For this review, take the finished solid that the model builds, in its own axes (mm). A direction names the side the tool comes from. Round coordinates to 2 decimals unless told otherwise and drop trailing zeros. Order: outer loops, then holes, each group sorted by start corner. A loop starts at its lowest first (then second) coordinate and runs counter-clockwise, first axis right, second up. Notation, with made-up numbers: (-17.75, 1.5) - (40.25, 1.5) arc R27 cw to (40.25, 40.5) - close; hole circle Ø4 at (68, 16.25). An arc over 180 degrees is marked (long way). Write each question's results on one line, items separated by ' | '. Start each with the question number.
(1) Take a section at A-A, the plane y = 9.5. Give the boundary of the cut face in (x, z), plus the area to 3 significant figures.
(2) Insertion check: pin 1 Ø5 at (y, z) = (-2.5, -6.5) entering from -X; pin 2 Ø4.5 at (x, z) = (29.5, -7.5) entering from -Y; pin 3 Ø1.7 at (x, y) = (30, -1.5) entering from -Z; pin 4 Ø4 at (x, z) = (22, -9) entering from -Y. Each pin has a flat end and moves straight along its axis. Give the tip position at first contact, or say it passes through.
(3) Draft analysis for pull direction Y (two halves, no side actions). For faces 5 (the flat face through (25.95, 0, -9)), 6 (the flat face through (29, 7.7, -8)), 7 (the flat face through (25.95, 9, -8)), state which applies: pulls with the +Y half, pulls with the -Y half, needs draft (parallel to the pull), parting line crosses it, or undercut.
(4) Take a section at B-B, the plane x = 30.25. Give the boundary of the cut face in (y, z), plus the area to 3 significant figures.
(5) Take a section at C-C, the plane z = -8.75. Give the boundary of the cut face in (x, y), plus the area to 3 significant figures.
(6) Take a section at D-D, the plane z = -5.75. Give the boundary of the cut face in (x, y), plus the area to 3 significant figures.
(7) For faces 1 (the flat face through (29, 0, -2.27)), 2 (the flat face through (25.95, -9, -8)), 3 (the flat face through (20, 8, -13.52)), 4 (the flat face through (24.95, 0, -7)), list the 3-axis set-ups (+Z, -Z, +X, -X, +Y, -Y) from which the entire face can be reached by the end or side of a thin tool; tool diameter is ignored.
(8) For L1, parallel to Y at x = 28.75, z = -12; L2, parallel to Z at x = 20.25, y = 6; L3, parallel to Z at x = 31.25, y = 1, list the stretches that pass through material, from the lowest coordinate up. Write a range as from..to.
```python
from build123d import *

# Parameters (mm, degrees)
PAD011_DEPTH = 5.65
SKETCH019_W  = 22.5
SKETCH019_H  = 14.7
PAD012_DEPTH = 1
PAD016_DEPTH = 6
FILLET_R     = 3


with BuildPart() as part:
    # Sketch018 → Pad011 (new body)
    with BuildSketch(Plane.YZ.offset(31.6)):
        Polygon((-6.6, -7.985767665), (-3.3, -2.27), (3.3, -2.27), (6.6, -7.985767665), (6.6, -15.52), (7.7, -15.52), (7.7, -0.82), (-7.7, -0.82), (-7.7, -15.52), (-6.6, -15.52), align=None)
    extrude(amount=-PAD011_DEPTH)

    # Sketch019 → Pad012 (new body)
    with BuildSketch(Plane(origin=(25.95, 0, 0), x_dir=(0, 1, 0), z_dir=(-1, 0, 0))):
        with Locations((0, 8.17)):
            Rectangle(SKETCH019_W, SKETCH019_H)
    extrude(amount=PAD012_DEPTH)

    # Sketch027 → Pad016 (new body)
    with BuildSketch(Plane(origin=(24.95, 0, 0), x_dir=(0, 1, 0), z_dir=(-1, 0, 0))):
        with BuildLine():
            Line((-11.25, 15.52), (11.25, 15.52))
            Line((11.25, 15.52), (11.25, 13.52))
            Line((11.25, 13.52), (4.0445515162, 13.52))
            ThreePointArc((4.0445515162, 13.52), (-1, 15.47), (-6.0445515162, 13.52))
            Line((-11.25, 13.52), (-6.0445515162, 13.52))
            Line((-11.25, 15.52), (-11.25, 13.52))
        make_face()
    extrude(amount=PAD016_DEPTH)

    # Fillet
    fillet_edges = [part.edges().sort_by_distance(p)[0] for p in [
        (24.95, -8.647276, -13.52),
        (24.95, 7.647276, -13.52),
    ]]
    fillet(fillet_edges, radius=FILLET_R)


solid = part.part
```
Results below:
1) outline: (18.95, -15.52) - (25.95, -15.52) - (25.95, -0.82) - (24.95, -0.82) - (24.95, -10.52) arc R3 cw to (21.95, -13.52) - (18.95, -13.52) - close | area: 28.6 mm^2
2) pin 1: stops at x = 24.95 | pin 2: stops at y = -7.7 | pin 3: stops at z = -2.27 | pin 4: passes through
3) face 5: undercut | face 6: pulls with the +Y half | face 7: needs draft
4) outline: (-7.7, -15.52) - (-6.6, -15.52) - (-6.6, -7.99) - (-3.3, -2.27) - (3.3, -2.27) - (6.6, -7.99) - (6.6, -15.52) - (7.7, -15.52) - (7.7, -0.82) - (-7.7, -0.82) - close | area: 70.3 mm^2
5) outline: (24.95, -11.25) - (25.95, -11.25) - (25.95, -7.7) - (31.6, -7.7) - (31.6, -6.6) - (25.95, -6.6) - (25.95, 6.6) - (31.6, 6.6) - (31.6, 7.7) - (25.95, 7.7) - (25.95, 11.25) - (24.95, 11.25) - close | area: 34.9 mm^2
6) outline: (24.95, -11.25) - (25.95, -11.25) - (25.95, -7.7) - (31.6, -7.7) - (31.6, -5.31) - (25.95, -5.31) - (25.95, 5.31) - (31.6, 5.31) - (31.6, 7.7) - (25.95, 7.7) - (25.95, 11.25) - (24.95, 11.25) - close | area: 49.5 mm^2
7) face 1: -Z, +X | face 2: +Z, -Z, +X, -Y | face 3: +Z, -X, +Y, -Y | face 4: +Z, -X
8) L1: y = -7.7..-6.6, 6.6..7.7 | L2: z = -15.52..-13.52 | L3: z = -2.27..-0.82
